Build history of the part. All positions in model axes, mm. A direction names the side the tool comes from. Round coordinates to 2 decimals unless told otherwise and drop trailing zeros. Write each loop counter-clockwise with the first axis right and the second up, starting at its lowest first coordinate (ties: lowest second). Pieces come first, ordered by that corner, then holes. Notation, with made-up numbers: M 53.5,87 L 112.5,87 A19 ccw 112.5,124 Z; hole C -9,85.5 d5. An arc over 180 degrees is marked long. Write item = value, one per line. Start each with the question number.
Q1. Pull direction Z, two halves, no side cores. Call faces 1 (the flat face through (41.589, 9.86, -95.845)), 2 (the flat face through (-1, 4, -124.24)), 3 (the flat face through (-35, 10, -99)): released by +Z, released by -Z, zero draft, split by the parting line, or undercut.
Q2. Drop flat-ended pins along their axis: P1, Ø2, axis at y = -4.5, z = -125, coming from the +X side; P2, Ø1, axis at x = -44.5, y = 9, coming from the +Z side; P3, Ø4, axis at x = 26.5, z = -117, coming from the -Y side; P4, Ø0.6, axis at x = 11, y = 15, coming from the +Z side. Give the stop position or say it passes through.
Q3. Band-saw the part on C-C on x = -28. Write the cut outline in (y, z).
Q4. Band-saw the part on B-B on y = -5.5. Write the cut outline in (x, z), plus the area to 3 significant figures.
Q5. Probe L1, parallel to X at y = 14, z = -122; L2, parallel to Y at x = 13, z = -114.5; L3, parallel to Z at x = -23, y = -9. List the from-to ranges inside material, lowest first.
Q6. Band-saw the part on A-A on z = -105. Write the cut outline in (x, y).
Q7. Band-saw the part on D-D on y = 10. State how many separate pieces and enclosed holes the cut face has, plus the area to 3 significant figures.
Q8. Tool access for faces 4 (the flat face through (-33, 10, -123)), 5 (the flat face through (44, 10, -97.24)), 6 (the flat face through (-1, 0, -111)), 7 (the flat face through (40, 10, -100.24)): list every direction of +Z, -Z, +X, -X, +Y, -Y with a clear straight run to the whole face (end or side of a thin tool).
```python
from build123d import *

# Parameters (mm, degrees)
EXTRUDE_1_DEPTH      = 20
SKETCH_2_W           = 200
SKETCH_2_H           = 1
EXTRUDE_2_DEPTH      = 20
SKETCH_3_R           = 1
EXTRUDE_3_DEPTH      = 100
SKETCH_4_W           = 70
SKETCH_4_H           = 15
CUT_EXTRUDE_1_DEPTH  = 150
CUT_EXTRUDE_START    = -150
CUT_EXTRUDE_2_DEPTH  = 150
EXTRUDE_4_DEPTH      = 20
SKETCH_7_W           = 70
SKETCH_7_H           = 15
CUT_EXTRUDE_3_DEPTH  = 50
SKETCH_8_W           = 18
SKETCH_8_H           = 15
CUT_EXTRUDE_4_DEPTH  = 50
SKETCH_9_W           = 18
SKETCH_9_H           = 15
CUT_EXTRUDE_5_DEPTH  = 50
SKETCH_10_W          = 241.24793126
SKETCH_10_H          = 101.321343747
CUT_EXTRUDE_6_DEPTH  = 50
SKETCH_11_W          = 124.388349514
SKETCH_11_H          = 45
EXTRUDE_5_DEPTH      = 10
CUT_EXTRUDE_7_DEPTH  = 200
EXTRUDE_6_DEPTH      = 124.5
CUT_EXTRUDE_8_DEPTH  = 134.5
SKETCH_15_W          = 13.694174757
SKETCH_15_H          = 51
SKETCH_15_W_2        = 13.805825243
CUT_EXTRUDE_9_DEPTH  = 40
CUT_EXTRUDE_10_DEPTH = 120
SKETCH_17_W          = 66
SKETCH_17_H          = 11
CUT_EXTRUDE_12_DEPTH = 120
SKETCH_18_W          = 3
SKETCH_18_H          = 51
CUT_EXTRUDE_13_DEPTH = 120
CUT_EXTRUDE_14_DEPTH = 6


with BuildPart() as part:
    # Sketch 1 → Extrude 1 (new body)
    with BuildSketch(Plane(origin=(0, 0, 0), x_dir=(1, 0, 0), z_dir=(0, 1, 0))):
        with BuildLine():
            Line((-42.194174757, 97.24017491), (-41, 94.488094488))
            ThreePointArc((-41, 94.488094488), (0, 103), (41, 94.488094488))
            Line((41, 94.488094488), (42.194174757, 97.24017491))
            ThreePointArc((42.194174757, 97.24017491), (0, 106), (-42.194174757, 97.24017491))
        make_face()
    extrude(amount=EXTRUDE_1_DEPTH)



with BuildPart() as body_2:
    # Sketch 2 → Extrude 2 (new body)
    with BuildSketch(Plane.XZ):
        with Locations((0, -0.5)):
            Rectangle(SKETCH_2_W, SKETCH_2_H)
    extrude(amount=-EXTRUDE_2_DEPTH)


with BuildPart() as part_1:
    add(part.part)

    add(body_2.part)  # Extrude 3 merges body 2
    # Sketch 3 → Extrude 3 (add)
    with BuildSketch(Plane(origin=(0, 0, -1), x_dir=(-1, 0, 0), z_dir=(0, 0, -1))):
        with Locations(Location((-39.194174757, 10, 0), (0, 0, 180))):
            Circle(SKETCH_3_R)
        with Locations(Location((39.194174757, 10, 0), (0, 0, 180))):
            Circle(SKETCH_3_R)
    extrude(amount=EXTRUDE_3_DEPTH)

    # Sketch 4 → Cut-Extrude 1 (cut)
    with BuildSketch(Plane(origin=(0, 0, -1), x_dir=(-1, 0, 0), z_dir=(0, 0, -1))):
        with Locations((0, 10)):
            Rectangle(SKETCH_4_W, SKETCH_4_H)
    extrude(amount=CUT_EXTRUDE_1_DEPTH, mode=Mode.SUBTRACT)

    # Sketch 5 → Cut-Extrude 2 (cut)
    with BuildSketch(Plane(origin=(0, 20, 0), x_dir=(1, 0, 0), z_dir=(0, 1, 0)).offset(CUT_EXTRUDE_START)):
        with BuildLine():
            Line((-49.057927096, 113.337024581), (-42.194174757, 97.24017491))
            ThreePointArc((-42.194174757, 97.24017491), (0, 106), (42.194174757, 97.24017491))
            Line((42.194174757, 97.24017491), (51.628141839, 112.189555316))
            ThreePointArc((51.628141839, 112.189555316), (1.407363629, 123.490812126), (-49.057927096, 113.337024581))
        make_face()
    extrude(amount=CUT_EXTRUDE_2_DEPTH, mode=Mode.SUBTRACT)

    # Sketch 6 → Extrude 4 (add)
    with BuildSketch(Plane.XZ):
        with BuildLine():
            Line((-42.194174757, -97.24017491), (-62.194174757, -97.24017491))
            Line((-62.194174757, -97.24017491), (-62.194174757, -122.24017491))
            Line((-62.194174757, -122.24017491), (62.194174757, -122.24017491))
            Line((62.194174757, -122.24017491), (62.194174757, -97.24017491))
            Line((62.194174757, -97.24017491), (42.194174757, -97.24017491))
            ThreePointArc((42.194174757, -97.24017491), (0, -106), (-42.194174757, -97.24017491))
        make_face()
    extrude(amount=-EXTRUDE_4_DEPTH)

    # Sketch 7 → Cut-Extrude 3 (cut)
    with BuildSketch(Plane(origin=(0, 0, -122.24017491), x_dir=(-1, 0, 0), z_dir=(0, 0, -1))):
        with Locations((0, 10)):
            Rectangle(SKETCH_7_W, SKETCH_7_H)
    extrude(amount=-CUT_EXTRUDE_3_DEPTH, mode=Mode.SUBTRACT)

    # Sketch 8 → Cut-Extrude 4 (cut)
    with BuildSketch(Plane.ZY.offset(62.194174757)):
        with Locations((-109.24017491, 10)):
            Rectangle(SKETCH_8_W, SKETCH_8_H)
    extrude(amount=-CUT_EXTRUDE_4_DEPTH, mode=Mode.SUBTRACT)

    # Sketch 9 → Cut-Extrude 5 (cut)
    with BuildSketch(Plane(origin=(62.194174757, 0, 0), x_dir=(0, 0, -1), z_dir=(1, 0, 0))):
        with Locations((109.24017491, 10)):
            Rectangle(SKETCH_9_W, SKETCH_9_H)
    extrude(amount=-CUT_EXTRUDE_5_DEPTH, mode=Mode.SUBTRACT)

    # Sketch 10 → Cut-Extrude 6 (cut)
    with BuildSketch(Plane(origin=(0, 20, 0), x_dir=(1, 0, 0), z_dir=(0, 1, 0))):
        with Locations((-3.693281443, 36.368377787)):
            Rectangle(SKETCH_10_W, SKETCH_10_H)
    extrude(amount=-CUT_EXTRUDE_6_DEPTH, mode=Mode.SUBTRACT)

    # Sketch 11 → Extrude 5 (add)
    with BuildSketch(Plane(origin=(0, 0, -122.24017491), x_dir=(-1, 0, 0), z_dir=(0, 0, -1))):
        with Locations((0, 10)):
            Rectangle(SKETCH_11_W, SKETCH_11_H)
    extrude(amount=EXTRUDE_5_DEPTH)

    # Sketch 12 → Cut-Extrude 7 (cut)
    with BuildSketch(Plane(origin=(62.194174757, 0, 0), x_dir=(0, 0, -1), z_dir=(1, 0, 0))):
        Polygon((122.24017491, 20), (132.24017491, 32.5), (122.24017491, 32.5), align=None)
        Polygon((122.24017491, 0), (132.24017491, -12.5), (122.24017491, -12.5), align=None)
    extrude(amount=-CUT_EXTRUDE_7_DEPTH, mode=Mode.SUBTRACT)

    # Sketch 13 → Extrude 6 (add)
    with BuildSketch(Plane(origin=(62.194174757, 0, 0), x_dir=(0, 0, -1), z_dir=(1, 0, 0))):
        Polygon((122.24017491, 0), (132.24017491, -12.5), (148.24017491, -12.5), (122.24017491, 20), align=None)
    extrude(amount=-EXTRUDE_6_DEPTH)

    # Sketch 14 → Cut-Extrude 8 (cut)
    with BuildSketch(Plane(origin=(62.194174757, 0, 0), x_dir=(0, 0, -1), z_dir=(1, 0, 0))):
        Polygon((122.24017491, 20), (132.24017491, 7.5), (132.24017491, 32.5), align=None)
    extrude(amount=-CUT_EXTRUDE_8_DEPTH, mode=Mode.SUBTRACT)

    # Sketch 15 → Cut-Extrude 9 (cut)
    with BuildSketch(Plane(origin=(0, 20, 0), x_dir=(1, 0, 0), z_dir=(0, 1, 0))):
        with Locations((55.347087379, 122.74017491)):
            Rectangle(SKETCH_15_W, SKETCH_15_H)
        with Locations((-55.402912622, 122.74017491)):
            Rectangle(SKETCH_15_W_2, SKETCH_15_H)
    extrude(amount=-CUT_EXTRUDE_9_DEPTH, mode=Mode.SUBTRACT)

    # Sketch 16 → Cut-Extrude 10 (cut)
    with BuildSketch(Plane.ZY.offset(48.5)):
        Polygon((-124.24017491, 14.298437881), (-144.078925215, -10.5), (-133.201424605, -10.5), (-124.24017491, 0.701562119), align=None)
    extrude(amount=-CUT_EXTRUDE_10_DEPTH, mode=Mode.SUBTRACT)

    # Sketch 17 → Cut-Extrude 12 (cut)
    with BuildSketch(Plane(origin=(0, 0, -124.24017491), x_dir=(-1, 0, 0), z_dir=(0, 0, -1))):
        with Locations((0, 10)):
            Rectangle(SKETCH_17_W, SKETCH_17_H)
    extrude(amount=-CUT_EXTRUDE_12_DEPTH, mode=Mode.SUBTRACT)

    # Sketch 18 → Cut-Extrude 13 (cut)
    with BuildSketch(Plane(origin=(0, 20, 0), x_dir=(1, 0, 0), z_dir=(0, 1, 0))):
        with Locations((-47, 122.74017491)):
            Rectangle(SKETCH_18_W, SKETCH_18_H)
        with Locations((47, 122.74017491)):
            Rectangle(SKETCH_18_W, SKETCH_18_H)
    extrude(amount=-CUT_EXTRUDE_13_DEPTH, mode=Mode.SUBTRACT)

    # Sketch 22 → Cut-Extrude 14 (cut)
    with BuildSketch(Plane(origin=(45.5, 0, 0), x_dir=(0, 0, -1), z_dir=(1, 0, 0))):
        Polygon((124.24017491, 14.298437881), (144.078925215, -10.5), (147.983269262, -7.376524762), (128.144518957, 17.421913119), align=None)
    extrude(amount=-CUT_EXTRUDE_14_DEPTH, mode=Mode.SUBTRACT)


solid = part_1.part
```
Conclusion:
q1.face_1 = released by +Z
q1.face_2 = undercut
q1.face_3 = zero draft
q2.P1 = 45.5
q2.P2 = -97.24
q2.P3 = 0
q2.P4 = -124.24
q3.outline = M -12.5,-148.24 L 20,-122.24 L 20,-99.12 L 17.5,-99.12 L 17.5,-122.24 L 15.5,-122.24 L 15.5,-124.24 L 14.3,-124.24 L -10.5,-144.08 L -10.5,-133.2 L 0.7,-124.24 L 4.5,-124.24 L 4.5,-122.24 L 2.5,-122.24 L 2.5,-99.12 L 0,-99.12 L 0,-122.24 L -12.5,-132.24 Z
q4.outline = M -45.5,-142.64 L 39.5,-142.64 L 39.5,-140.08 L -45.5,-140.08 Z; M -45.5,-129.2 L 45.5,-129.2 L 45.5,-126.64 L -45.5,-126.64 Z
q4.area = 451 mm^2
q5.L1 = -45.5 to -35, 35 to 45.5
q5.L2 = 0 to 2.5, 17.5 to 20
q5.L3 = -145.44 to -142.88, -132 to -129.44
q6.outline = M -45.5,0 L 45.5,0 L 45.5,2.5 L -45.5,2.5 Z; M -45.5,17.5 L 45.5,17.5 L 45.5,20 L -45.5,20 Z
q7.separate_pieces = 5
q7.enclosed_holes = 0
q7.area = 469 mm^2
q8.face_4 = +Z
q8.face_5 = +Z, +X, +Y, -Y
q8.face_6 = +Z, +X, -X, -Y
q8.face_7 = +X, -X
